Autodesk Inventor part; units mm, degrees
ref_plane "YZ Plane" through (0, 0, 0) normal (1, 0, 0) x (0, 1, 0)
ref_plane "XZ Plane" through (0, 0, 0) normal (0, 1, 0) x (-1, 0, 0)
ref_plane "XY Plane" through (0, 0, 0) normal (0, 0, 1) x (1, 0, 0)
sketch "Sketch1" plane through (0, 0, 0) normal (0, 1, 0) x (-1, 0, 0)
  line L0 (60, 8) -> (-60, 8)
  line L1 (-60, 8) -> (-60, -8)
  line L2 (-60, -8) -> (60, -8)
  line L3 (60, -8) -> (60, 8)
  line L4 (60, 8) -> (-60, -8) construction
  line L5 (-60, 8) -> (60, -8) construction
  point P0 (0, 0)
  dimension "d0" = 16
  dimension "d1" = 120
extrude "Extrusion1" add sketch "Sketch1" along normal blind 10
hole "Hole1" at (0, 10, 0) direction (0, -1, 0) diameter 7.142 depth 25.4 counterbore diameter 11.113 counterbore depth 6.35
sketch "Sketch2" plane through (0, 10, 0) normal (0, 1, 0) x (1, 0, 0)
  circle A0 centre (15, 0) radius 2.75
  circle A1 centre (45, 0) radius 2.75
  circle A2 centre (-15, 0) radius 2.75
  circle A3 centre (-45, 0) radius 2.75
  point P0 (0, 0)
  dimension "d15" = 5.5
  dimension "d16" = 15
  dimension "d17" = 30
  dimension "d18" = 5.5
  dimension "d19" = 15
  dimension "d20" = 5.5
  dimension "d21" = 30
  dimension "d22" = 5.5
extrude "Extrusion2" cut sketch "Sketch2" against normal up to next
sketch "Sketch6" plane through (-60, 0, 8) normal (0, 0, 1) x (1, 0, 0)
  line L0 (120, 10) -> (0, 10)
  line L1 (0, 0) -> (120, 0)
  line L2 (7.5, 10) -> (22.5, 10)
  line L3 (22.5, 10) -> (22.5, 0)
  line L4 (22.5, 0) -> (7.5, 0)
  line L5 (7.5, 0) -> (7.5, 10)
  line L6 (0, 0) -> (0, 10)
  line L7 (0, 10) -> (120, 10)
  line L8 (37.5, 10) -> (52.5, 10)
  line L9 (52.5, 10) -> (52.5, 0)
  line L10 (52.5, 0) -> (37.5, 0)
  line L11 (37.5, 0) -> (37.5, 10)
  line L12 (67.5, 10) -> (82.5, 10)
  line L13 (82.5, 10) -> (82.5, 0)
  line L14 (82.5, 0) -> (67.5, 0)
  line L15 (67.5, 0) -> (67.5, 10)
  line L16 (97.5, 10) -> (112.5, 10)
  line L17 (112.5, 10) -> (112.5, 0)
  line L18 (112.5, 0) -> (97.5, 0)
  line L19 (97.5, 0) -> (97.5, 10)
  line L20 (127.5, 10) -> (142.5, 10)
  line L21 (142.5, 10) -> (142.5, 0)
  line L22 (142.5, 0) -> (127.5, 0)
  line L23 (127.5, 0) -> (127.5, 10)
  point P0 (60, 0)
  point P1 (150, 10)
  point P2 (150, 0)
  dimension "d33" = 15
  dimension "d34" = 7.5
  dimension "d35" = 15
  dimension "d36" = 15
  dimension "d37" = 15
  dimension "d38" = 15
  dimension "d39" = 15
  dimension "d40" = 15
  dimension "d41" = 15
  dimension "d42" = 15
extrude "Extrusion5" add sketch "Sketch6" along normal blind 40 contours L17 L1 L19 L0 | L13 L1 L15 L0 | L9 L1 L11 L0 | L3 L1 L5 L0
sketch "Sketch7" plane through (0, 10, 0) normal (0, 1, 0) x (1, 0, 0)
  circle A0 centre (-45, -41) radius 2.75
  circle A1 centre (-45, 0) radius 2.75
  line L0 (-52.5, -8) -> (-52.5, -48)
  circle A2 centre (-15, -41) radius 2.75
  circle A3 centre (15, -41) radius 2.75
  circle A4 centre (45, -41) radius 2.75
  circle A5 centre (75, -41) radius 2.75
  point P0 (0, 0)
  dimension "d45" = 5.5
  dimension "d46" = 41
  dimension "d47" = 7.5
  dimension "d48" = 5.5
  dimension "d49" = 5.5
  dimension "d50" = 5.5
  dimension "d51" = 5.5
extrude "Extrusion6" cut sketch "Sketch7" against normal up to next contours A0 | A2 | A3 | A4 | A5
fillet "Fillet1" radius 2 20 edges at (-52.5, 5, 48) (-37.5, 5, 48) (-22.5, 5, 48) (-7.5, 5, 48) (7.5, 5, 48) (22.5, 5, 48) (37.5, 5, 48) (52.5, 5, 48) (-60, 5, 8) (-60, 5, -8) (-52.5, 5, 8) (-37.5, 5, 8) (-22.5, 5, 8) (7.5, 5, 8) (37.5, 5, 8) (52.5, 5, 8) (22.5, 5, 8) (-7.5, 5, 8) (60, 5, 8) (60, 5, -8)
properties part number "FlowmeterMountThorX4"
Work out the finished part from the listing and answer in its coordinate system (mm). A direction names the side the tool comes from. Round coordinates to 2 decimals unless told otherwise and drop trailing zeros. Order: outer loops, then holes, each group sorted by start corner. A loop starts at its lowest first (then second) coordinate and runs counter-clockwise, first axis right, second up.
Q1. Given pin 1 Ø3 at (x, y) = (29, 5.5) entering from +Z; pin 2 Ø5.5 at (x, z) = (0, -2.5) entering from +Y; pin 3 Ø6 at (y, z) = (7, 11.5) entering from +X, each flat-ended and moving along its own axis, determine where each tip first touches the part or whether it passes through.
Solution:
pin 1: stops at z = 8
pin 2: stops at y = 3.65
pin 3: stops at x = 53.18
Q2. A tool of negligible diameter and unlimited length cuts with its end or side. For faces 1 (the flat face through (56, 5, 8)), 2 (the cylindrical face through (42.253, 5.07, -0.121)), 3 (the flat face through (0, 5, 8)), from which of +Z, -Z, +X, -X, +Y, -Y can it reach the whole face along a straight path? Write none if from no direction.
Solution:
face 1: +Z, +X, +Y, -Y
face 2: +Y, -Y
face 3: +Z, +Y, -Y
Q3. A cutting plane is placed at D-D, the plane z = 41. Count the separate pieces of the cut face and the enclosed holes in it, then the cut area to 3 significant figures.
Solution:
separate pieces: 8
enclosed holes: 0
area: 380 mm2
Q4. A cutting plane is placed at B-B, the plane z = 0. Determine the outline of the cut face in (x, y).
Solution:
outline: (-60, 0) - (-47.75, 0) - (-47.75, 10) - (-60, 10) - close; (-42.25, 0) - (-17.75, 0) - (-17.75, 10) - (-42.25, 10) - close; (-12.25, 0) - (-3.57, 0) - (-3.57, 3.65) - (-5.56, 3.65) - (-5.56, 10) - (-12.25, 10) - close; (3.57, 0) - (12.25, 0) - (12.25, 10) - (5.56, 10) - (5.56, 3.65) - (3.57, 3.65) - close; (17.75, 0) - (42.25, 0) - (42.25, 10) - (17.75, 10) - close; (47.75, 0) - (60, 0) - (60, 10) - (47.75, 10) - close
Q5. The mould has two halves that part along Z. Classify faces 4 (the cylindrical face through (12.253, 5.07, -0.121)), 5 (the cylindrical face through (-36.93, 4.93, 8.6)), 6 (the flat face through (7.5, 5, 28)): pulls with the +Z half, pulls with the -Z half, needs draft (parallel to the pull), parting line crosses it, or undercut.
Solution:
face 4: undercut
face 5: pulls with the +Z half
face 6: needs draft
Q6. A cutting plane is placed at C-C, the plane z = 31. Determine the outline of the cut face in (x, y).
Solution:
outline: (-52.5, 0) - (-37.5, 0) - (-37.5, 10) - (-52.5, 10) - close; (-22.5, 0) - (-7.5, 0) - (-7.5, 10) - (-22.5, 10) - close; (7.5, 0) - (22.5, 0) - (22.5, 10) - (7.5, 10) - close; (37.5, 0) - (52.5, 0) - (52.5, 10) - (37.5, 10) - close
Q7. A cutting plane is placed at A-A, the plane x = -15. Determine the outline of the cut face in (y, z).
Solution:
outline: (0, -8) - (10, -8) - (10, -2.75) - (0, -2.75) - close; (0, 2.75) - (10, 2.75) - (10, 38.25) - (0, 38.25) - close; (0, 43.75) - (10, 43.75) - (10, 48) - (0, 48) - close
Q8. Find the intervals of material crossed by line 1 along X through (y, z) = (6, 15); line 2 along Z through (x, y) = (-15, 5); line 3 along X through (y, z) = (7.5, 0), in increasing order.
Solution:
line 1: x = -52.5 to -37.5, -22.5 to -7.5, 7.5 to 22.5, 37.5 to 52.5
line 2: z = -8 to -2.75, 2.75 to 38.25, 43.75 to 48
line 3: x = -60 to -47.75, -42.25 to -17.75, -12.25 to -5.56, 5.56 to 12.25, 17.75 to 42.25, 47.75 to 60
